Input: dimensioned drawing with shaded views. Units: mm. Origin: part minimum x, y, z. Give positions to 0.01 mm unless a question says otherwise; leave off trailing zeros. Loops run counter-clockwise (first coordinate to the right, second up) from the corner with the lowest first, then second, coordinate; pieces in that order, holes last. Notation, with made-up numbers: (-29.75, 4) -> (-9.75, 4) arc R20 ccw to (-9.75, 43) -> close; hole circle Ø3 at (-23, 37). An arc over 180 degrees is marked (long way). Answer as a JSON object with one key per item and string values.
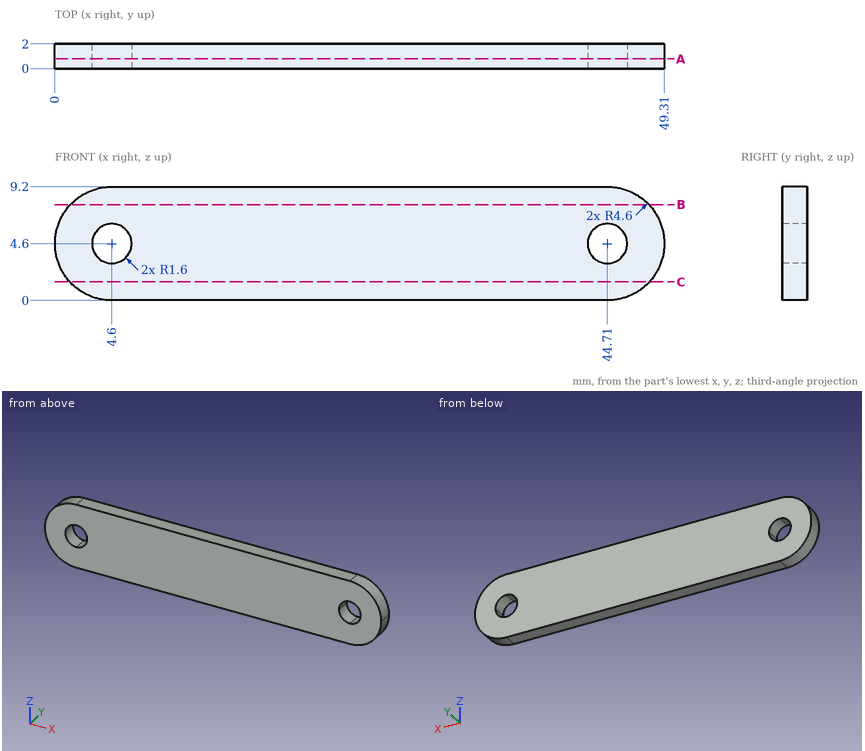
Q1. Section C-C, the plane z = 1.5. Return the cut outline in (x, y).
Evaluation:
{"outline": "(1.2, 0) -> (48.11, 0) -> (48.11, 2) -> (1.2, 2) -> close"}
Q2. Section B-B, the plane z = 7.75. Return the cut outline in (x, y), then the cut area to 3 significant figures.
Evaluation:
{"outline": "(1.25, 0) -> (48.06, 0) -> (48.06, 2) -> (1.25, 2) -> close", "area": "93.6 mm2"}
Q3. Section A-A, the plane y = 0.8. Return the cut outline in (x, z).
Evaluation:
{"outline": "(4.6, 0) -> (44.71, 0) arc R4.6 ccw to (44.71, 9.2) -> (4.6, 9.2) arc R4.6 ccw to start; hole circle Ø3.2 at (4.6, 4.6); hole circle Ø3.2 at (44.71, 4.6)"}
Q4. Ray query, line 1 along X through (y, z) = (1.2, 3.25); line 2 along X through (y, z) = (0.95, 4.5); line 3 along Z through (x, y) = (45.5, 1.85). Return the intervals inside material, ascending.
Evaluation:
{"line 1": "x = 0.2 to 3.74, 5.46 to 43.85, 45.57 to 49.11", "line 2": "x = 0 to 3, 6.2 to 43.11, 46.31 to 49.31", "line 3": "z = 0.07 to 3.21, 5.99 to 9.13"}
